Autodesk Inventor part; units mm, degrees
ref_plane "YZ Plane" through (0, 0, 0) normal (1, 0, 0) x (0, 1, 0)
ref_plane "XZ Plane" through (0, 0, 0) normal (0, 1, 0) x (-1, 0, 0)
ref_plane "XY Plane" through (0, 0, 0) normal (0, 0, 1) x (1, 0, 0)
sketch "Sketch1" plane through (0, 0, 0) normal (0, 0, 1) x (1, 0, 0)
  circle A0 centre (0, 0) radius 4.7625 construction
  line L0 (2.7496, 4.7625) -> (5.4993, 0)
  line L1 (5.4993, 0) -> (2.7496, -4.7625)
  line L2 (2.7496, -4.7625) -> (-2.7496, -4.7625)
  line L3 (-2.7496, -4.7625) -> (-5.4993, 0)
  line L4 (-5.4993, 0) -> (-2.7496, 4.7625)
  line L5 (-2.7496, 4.7625) -> (2.7496, 4.7625)
  point P0 (0, 4.7625)
  dimension "d0" = 9.525
extrude "Extrusion1" add sketch "Sketch1" along normal blind 3.175
sketch "Sketch2" plane through (0, 0, 3.175) normal (0, 0, 1) x (1, 0, 0)
  point P0 (0, 0)
hole "Hole1" at (0, 0, 3.175) direction (0, 0, -1) diameter 3.937 end through all
sketch "Sketch3" plane through (0, 0, 0) normal (1, 0, 0) x (0, 1, 0)
  line L0 (-4.7625, 3.175) -> (0, 3.175)
  line L1 (-4.7625, 0) -> (0, 0)
  line L2 (-4.7625, 3.175) -> (-6.7124, 3.175)
  line L3 (-6.7124, 3.175) -> (-6.7124, 2.0492)
  line L4 (-6.7124, 2.0492) -> (-4.7625, 3.175)
  line L5 (-4.7625, 0) -> (-6.7124, 0)
  line L6 (-6.7124, 0) -> (-6.7124, 1.1258)
  line L7 (-6.7124, 1.1258) -> (-4.7625, 0)
  line L8 (0, -0.3175) -> (0, 4.1275)
  dimension "d10" = 30
  dimension "d11" = 30
revolve "Revolution1" cut sketch "Sketch3" angle 360 about axis through (0, 0, -10) along (0, 0, 1)
sketch "Sketch4" plane through (0, 0, 3.175) normal (0, 0, 1) x (1, 0, 0)
  arc A0 (4.1244, -2.3813) -> (4.1244, 2.3813) centre (0, 0) ccw
  arc A1 (4.1244, 2.3813) -> (0, 4.7625) centre (0, 0) ccw
  arc A2 (0, 4.7625) -> (-4.1244, 2.3812) centre (0, 0) ccw
  arc A3 (-4.1244, 2.3812) -> (-4.1244, -2.3813) centre (0, 0) ccw
  arc A4 (-4.1244, -2.3813) -> (0, -4.7625) centre (0, 0) ccw
  arc A5 (0, -4.7625) -> (4.1244, -2.3813) centre (0, 0) ccw
  circle A6 centre (0, 0) radius 1.9685
  circle A7 centre (0, 0) radius 4.5085
  dimension "d16" = 0.254
extrude "Extrusion2" add sketch "Sketch4" along normal blind 1.27 contours A7
fillet "Fillet1" radius 1.905 1 edges at (-4.5085, 0, 4.445)
equation "\"d10\" = d11"
properties part number "PWTR-0034"
Part model, mm, in its own coordinate system. Give positions to 0.01 mm unless a question says otherwise; leave off trailing zeros. Order: outer loops, then holes, each group sorted by start corner. A loop starts at its lowest first (then second) coordinate and runs counter-clockwise, first axis right, second up. Notation, with made-up numbers: (88, 19) - (119, 19) arc R25 ccw to (119, 34) - close; hole circle Ø8 at (68.25, -36.75). An arc over 180 degrees is marked (long way). One line per question, with ' | ' between items.
1. Drop a flat-ended pin along its axis: P1, Ø1, axis at x = -1.5, z = 4, coming from the +Y side. Give the stop position or say it passes through.
Filled in:
P1: y = 4.13
2. Drill centre lines: probe 1 along Y at (x, z) = (0, 1.65); probe 2 along Z at (x, y) = (-1.5, 4.5) (3 decimals); probe 3 along X at (y, z) = (1.25, 2.7). Where is each one in solid material? Low to high.
Filled in:
probe 1: -4.76 to -1.97, 1.97 to 4.76 | probe 2: 0 to 3.175 | probe 3: -4.78 to -1.52, 1.52 to 4.78
3. Band-saw the part on A-A on z = 0.9. List the corners of the cut face in (x, y).
Filled in:
outline: (-5.5, 0) - (-2.75, -4.76) - (2.75, -4.76) - (5.5, 0) - (2.75, 4.76) - (-2.75, 4.76) - close; hole circle Ø3.94 at (0, 0)
